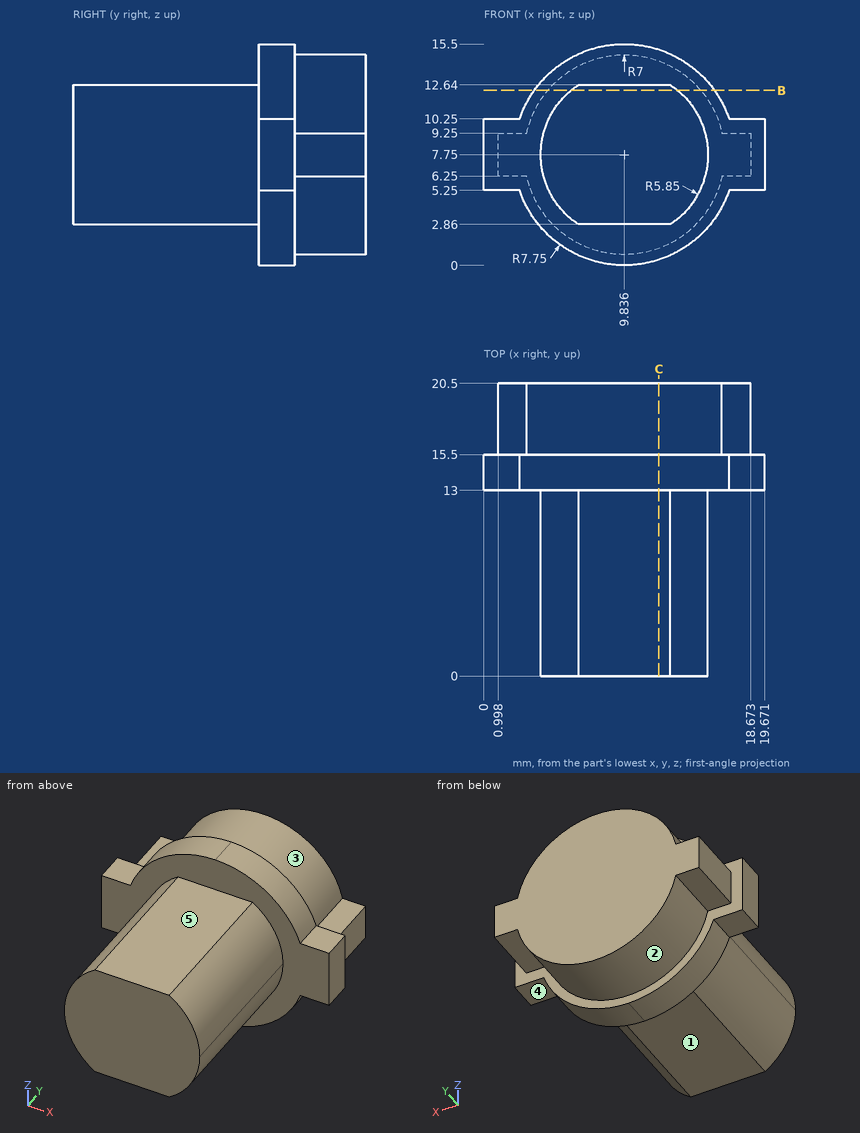
Study the drawing (mm; zero at the part's minimum x, y, z) and answer. A direction names the side the tool comes from. Round coordinates to 2 decimals unless told otherwise and drop trailing zeros. Loops run counter-clockwise (first coordinate to the right, second up) from the corner with the lowest first, then second, coordinate; pieces in that order, holes last.
Q1. Which of the six approach directions +Z, -Z, +X, -X, +Y, -Y give full straight-line access (tool end or side, diameter ignored) to the marked faces 1, 2, 3, 4 and 5?
Q2. Find the intervals of material crossed by line 1 (Z direction, x = 17, y = 17.25); line 2 (Y direction, x = 4.5, z = 12.75); line 3 (Z direction, x = 7.5, y = 6.5), in increasing order.
Q3. Given pin 1 Ø2 at (x, y) = (18, 14.5) entering from -Z (1 decimal); pin 2 Ø3 at (x, y) = (18.5, 14) entering from +Z (1 decimal); pin 3 Ø5 at (x, y) = (9.5, 4) entering from +Z; pin 4 Ø6 at (y, z) = (11.5, 12.5) entering from -X, each flat-ended and moving along its own axis, determine where each tip first touches the part or whether it passes through.
Q4. Section C-C, the plane x = 12.25 is taken. Determine the outline of the cut face in (y, z) (1 decimal).
Q5. Section B-B, the plane z = 12.25 is taken. Determine the outline of the cut face in (x, y) (1 decimal).
Completed:
1. face 1: -Z, +X, -X, -Y
1. face 2: -Z, +Y
1. face 3: +Z, +Y
1. face 4: -Z, +X, +Y, -Y
1. face 5: +Z, +X, -X, -Y
2. line 1: z = 6.25 to 9.25
2. line 2: y = 13 to 15.5
2. line 3: z = 2.86 to 12.64
3. pin 1: stops at z = 4.8
3. pin 2: stops at z = 10.7
3. pin 3: stops at z = 12.64
3. pin 4: stops at x = 0
4. outline: (0, 2.9) - (13, 2.9) - (13, 0.4) - (15.5, 0.4) - (15.5, 1.2) - (20.5, 1.2) - (20.5, 14.3) - (15.5, 14.3) - (15.5, 15.1) - (13, 15.1) - (13, 12.6) - (0, 12.6) - close
5. outline: (3.5, 13) - (6.1, 13) - (6.1, 0) - (13.6, 0) - (13.6, 13) - (16.1, 13) - (16.1, 15.5) - (15.2, 15.5) - (15.2, 20.5) - (4.5, 20.5) - (4.5, 15.5) - (3.5, 15.5) - close
